For this review, take the finished solid that the model builds, in its own axes (mm). A direction names the side the tool comes from. Round coordinates to 2 decimals unless told otherwise and drop trailing zeros. Write each loop counter-clockwise with the first axis right and the second up, starting at its lowest first coordinate (ties: lowest second). Pieces come first, ordered by that corner, then holes. Notation, with made-up numbers: M -6,14 L 10,14 A11 cw 10,18 Z; hole C -5,-15.5 d3. An arc over 180 degrees is marked long. Answer in a Markdown table with one row per item.
```python
from build123d import *

# Parameters (mm, degrees)
F1_DEPTH = 1.5
F2_DEPTH = 3.5
F3_R     = 1.49999
F5_DEPTH = 2


# Not quite as in the source:
# - a fillet or chamfer is up to 0.001 mm smaller than in the source, because OpenCascade refuses the exact size


with BuildPart() as f1:
    # F0 (on Top) → F1 (new body)
    with BuildSketch(Plane.XY):
        with BuildLine():
            Line((15.5, -0.9), (15.5, 0.9))
            ThreePointArc((15.5, 0.9), (14.4748737342, 3.3748737342), (12, 4.4))
            Line((12, 4.4), (-12, 4.4))
            ThreePointArc((-12, 4.4), (-14.4748737342, 3.3748737342), (-15.5, 0.9))
            Line((-15.5, 0.9), (-15.5, -0.9))
            ThreePointArc((-15.5, -0.9), (-14.4748737342, -3.3748737342), (-12, -4.4))
            Line((-12, -4.4), (12, -4.4))
            ThreePointArc((12, -4.4), (14.4748737342, -3.3748737342), (15.5, -0.9))
        make_face()
        with BuildLine():
            ThreePointArc((13.5, -0.9), (13.0606601718, -1.9606601718), (12, -2.4))
            Line((12, -2.4), (-12, -2.4))
            ThreePointArc((-12, -2.4), (-13.0606601718, -1.9606601718), (-13.5, -0.9))
            Line((-13.5, -0.9), (-13.5, 0.9))
            ThreePointArc((-13.5, 0.9), (-13.0606601718, 1.9606601718), (-12, 2.4))
            Line((-12, 2.4), (12, 2.4))
            ThreePointArc((12, 2.4), (13.0606601718, 1.9606601718), (13.5, 0.9))
            Line((13.5, 0.9), (13.5, -0.9))
        make_face(mode=Mode.SUBTRACT)
        with BuildLine():
            Line((-12, -2.4), (12, -2.4))
            ThreePointArc((12, -2.4), (13.0606601718, -1.9606601718), (13.5, -0.9))
            Line((13.5, -0.9), (13.5, 0.9))
            ThreePointArc((13.5, 0.9), (13.0606601718, 1.9606601718), (12, 2.4))
            Line((12, 2.4), (-12, 2.4))
            ThreePointArc((-12, 2.4), (-13.0606601718, 1.9606601718), (-13.5, 0.9))
            Line((-13.5, 0.9), (-13.5, -0.9))
            ThreePointArc((-13.5, -0.9), (-13.0606601718, -1.9606601718), (-12, -2.4))
        make_face()
        with BuildLine():
            ThreePointArc((12, 1.6), (12.4949747468, 1.3949747468), (12.7, 0.9))
            Line((12.7, 0.9), (12.7, -0.9))
            ThreePointArc((12.7, -0.9), (12.4949747468, -1.3949747468), (12, -1.6))
            Line((12, -1.6), (-12, -1.6))
            ThreePointArc((-12, -1.6), (-12.4949747468, -1.3949747468), (-12.7, -0.9))
            Line((-12.7, -0.9), (-12.7, 0.9))
            ThreePointArc((-12.7, 0.9), (-12.4949747468, 1.3949747468), (-12, 1.6))
            Line((-12, 1.6), (12, 1.6))
        make_face(mode=Mode.SUBTRACT)
        with BuildLine():
            Line((12.7, -0.9), (12.7, 0.9))
            ThreePointArc((12.7, 0.9), (12.4949747468, 1.3949747468), (12, 1.6))
            Line((12, 1.6), (-12, 1.6))
            ThreePointArc((-12, 1.6), (-12.4949747468, 1.3949747468), (-12.7, 0.9))
            Line((-12.7, 0.9), (-12.7, -0.9))
            ThreePointArc((-12.7, -0.9), (-12.4949747468, -1.3949747468), (-12, -1.6))
            Line((-12, -1.6), (12, -1.6))
            ThreePointArc((12, -1.6), (12.4949747468, -1.3949747468), (12.7, -0.9))
        make_face()
    extrude(amount=F1_DEPTH)

    # F0 (on Top) → F2 (join)
    with BuildSketch(Plane.XY):
        with BuildLine():
            Line((-12, -2.4), (12, -2.4))
            ThreePointArc((12, -2.4), (13.0606601718, -1.9606601718), (13.5, -0.9))
            Line((13.5, -0.9), (13.5, 0.9))
            ThreePointArc((13.5, 0.9), (13.0606601718, 1.9606601718), (12, 2.4))
            Line((12, 2.4), (-12, 2.4))
            ThreePointArc((-12, 2.4), (-13.0606601718, 1.9606601718), (-13.5, 0.9))
            Line((-13.5, 0.9), (-13.5, -0.9))
            ThreePointArc((-13.5, -0.9), (-13.0606601718, -1.9606601718), (-12, -2.4))
        make_face()
        with BuildLine():
            ThreePointArc((12, 1.6), (12.4949747468, 1.3949747468), (12.7, 0.9))
            Line((12.7, 0.9), (12.7, -0.9))
            ThreePointArc((12.7, -0.9), (12.4949747468, -1.3949747468), (12, -1.6))
            Line((12, -1.6), (-12, -1.6))
            ThreePointArc((-12, -1.6), (-12.4949747468, -1.3949747468), (-12.7, -0.9))
            Line((-12.7, -0.9), (-12.7, 0.9))
            ThreePointArc((-12.7, 0.9), (-12.4949747468, 1.3949747468), (-12, 1.6))
            Line((-12, 1.6), (12, 1.6))
        make_face(mode=Mode.SUBTRACT)
        with BuildLine():
            Line((12.7, -0.9), (12.7, 0.9))
            ThreePointArc((12.7, 0.9), (12.4949747468, 1.3949747468), (12, 1.6))
            Line((12, 1.6), (-12, 1.6))
            ThreePointArc((-12, 1.6), (-12.4949747468, 1.3949747468), (-12.7, 0.9))
            Line((-12.7, 0.9), (-12.7, -0.9))
            ThreePointArc((-12.7, -0.9), (-12.4949747468, -1.3949747468), (-12, -1.6))
            Line((-12, -1.6), (12, -1.6))
            ThreePointArc((12, -1.6), (12.4949747468, -1.3949747468), (12.7, -0.9))
        make_face()
    extrude(amount=F2_DEPTH)

    # F3 (radius 1.5 in the source; OpenCascade refuses exactly that, so slightly less here)
    f3_edges = [f1.edges().sort_by_distance(p)[0] for p in [
        (0, -4.4, 0),
        (-14.474874, -3.374874, 0),
        (-15.5, 0, 0),
        (14.474874, -3.374874, 0),
        (15.5, 0, 0),
        (14.474874, 3.374874, 0),
        (0, 4.4, 0),
        (-14.474874, 3.374874, 0),
    ]]
    fillet(f3_edges, radius=F3_R)

    # F4 (on face) → F5 (join, through all)
    with BuildSketch(Plane.XY.offset(3.5)):
        with BuildLine():
            ThreePointArc((-6.1542230954, -2.4), (-6.0387434053, -1.8553793215), (-6, -1.3))
            ThreePointArc((-6, -1.3), (-6.6773900574, 0.9271648276), (-8.4801315846, 2.4))
            Line((-8.4801315846, 2.4), (-11.5198684154, 2.4))
            ThreePointArc((-11.5198684154, 2.4), (-12.6603120365, 1.6870955573), (-13.5, 0.6364916731))
            Line((-13.5, 0.6364916731), (-13.5, -0.9))
            ThreePointArc((-13.5, -0.9), (-13.0606601718, -1.9606601718), (-12, -2.4))
            Line((-12, -2.4), (-6.1542230954, -2.4))
        make_face()
        with BuildLine():
            Line((-11.5198684154, 2.4), (-8.4801315846, 2.4))
            ThreePointArc((-8.4801315846, 2.4), (-10, 2.7), (-11.5198684154, 2.4))
        make_face()
        with BuildLine():
            Line((3.8157568057, 2.4), (-3.8157568057, 2.4))
            ThreePointArc((-3.8157568057, 2.4), (-3.6723969913, -0.3854022638), (-1.7435595774, -2.4))
            Line((-1.7435595774, -2.4), (1.7435595774, -2.4))
            ThreePointArc((1.7435595774, -2.4), (3.3892652825, -0.9243542184), (4, 1.2))
            ThreePointArc((4, 1.2), (3.9536709033, 1.8070307971), (3.8157568057, 2.4))
        make_face()
        with BuildLine():
            Line((1.7435595774, -2.4), (-1.7435595774, -2.4))
            ThreePointArc((-1.7435595774, -2.4), (0, -2.8), (1.7435595774, -2.4))
        make_face()
        with BuildLine():
            ThreePointArc((11.5198684154, 2.4), (10, 2.7), (8.4801315846, 2.4))
            Line((8.4801315846, 2.4), (11.5198684154, 2.4))
        make_face()
    extrude(amount=-F5_DEPTH)


solid = f1.part
```
Q1. Take a section at A-A (z = 0.6). State the section outline as (x, y) points.
Found:
| item | result |
|---|---|
| outline | M -15.2,-0.9 A3.2 ccw -12,-4.1 L 12,-4.1 A3.2 ccw 15.2,-0.9 L 15.2,0.9 A3.2 ccw 12,4.1 L -12,4.1 A3.2 ccw -15.2,0.9 Z |
Q2. For probe 1 along Z at (x, y) = (14, 1); probe 2 along Y at (x, z) = (-7, 1.6); probe 3 along Y at (x, z) = (11, 1.4), list the stretches that pass through material, from the lowest coordinate up.
Found:
| item | result |
|---|---|
| probe 1 | 0 to 1.5 |
| probe 2 | -2.4 to 2.4 |
| probe 3 | -4.4 to 4.4 |
Q3. Insertion check: P1, Ø1.5, axis at y = 3, z = 2, coming from the -X side; P2, Ø1.6, axis at x = 9, z = 2.5, coming from the -Y side; P3, Ø0.5, axis at y = 0, z = 3, coming from the +X side. Each pin has a flat end and moves straight along its axis. Give the tip position at first contact, or say it passes through.
Found:
| item | result |
|---|---|
| P1 | x = -15.14 |
| P2 | y = -2.4 |
| P3 | x = 13.5 |
Q4. Take a section at D-D (z = 1.95). State the section outline as (x, y) points, then the cut area to 3 significant figures.
Found:
| item | result |
|---|---|
| outline | M -13.5,-0.9 A1.5 ccw -12,-2.4 L -1.74,-2.4 A4 ccw 1.74,-2.4 L 12,-2.4 A1.5 ccw 13.5,-0.9 L 13.5,0.9 A1.5 ccw 12,2.4 L 11.52,2.4 A4 ccw 8.48,2.4 L -8.48,2.4 A4 ccw -11.52,2.4 L -12,2.4 A1.5 ccw -13.5,0.9 Z |
| area | 130 mm² |
Q5. Machinability: for faces 1 (the face through (-13.5, 0, 2)), 2 (the face through (7, -2.4, 2)), 3 (the face through (-13.07, -1.95, 2.49)), 4 (the face through (13.07, 1.95, 2.49)), 5 (the face through (0, 2.4, 2)), which of the approach directions +Z, -Z, +X, -X, +Y, -Y give a long, thin tool a straight path to every point of the face, cutting with its end or side? Answer none if there is none.
Found:
| item | result |
|---|---|
| face 1 | +Z, -X, +Y, -Y |
| face 2 | +Z, +X, -Y |
| face 3 | +Z, -X, -Y |
| face 4 | +Z, +X, +Y |
| face 5 | +Z, +Y |
